from build123d import *

# Parameters (mm, degrees)
SALIENTE_EXTRUIR1_DEPTH = 2
SALIENTE_EXTRUIR2_DEPTH = 100
CROQUIS3_W              = 58.7
CROQUIS3_H              = 38.2
CROQUIS3_R              = 1.5
CROQUIS3_W_2            = 38.8
CROQUIS3_H_2            = 35.8
CORTAR_EXTRUIR1_DEPTH   = 1
CROQUIS4_W              = 38.8
CROQUIS4_H              = 35.8
CORTAR_EXTRUIR2_DEPTH   = 12
CROQUIS5_W              = 58.7
CROQUIS5_H              = 38.2
CROQUIS5_R              = 1.5
CORTAR_EXTRUIR3_DEPTH   = 3
CROQUIS6_R              = 1
SALIENTE_EXTRUIR3_DEPTH = 3.4
CROQUIS8_R              = 1
CORTAR_EXTRUIR5_DEPTH   = 4
CORTAR_EXTRUIR6_DEPTH   = 0.6


with BuildPart() as part:
    # Croquis1 → Saliente-Extruir1 (new body)
    with BuildSketch(Plane(origin=(0, 0, 0), x_dir=(1, 0, 0), z_dir=(0, 1, 0))):
        with BuildLine():
            Line((-121.24355653, -10), (-69.282032303, -100))
            ThreePointArc((-69.282032303, -100), (-61.961524227, -107.320508076), (-51.961524227, -110))
            Line((-51.961524227, -110), (51.961524227, -110))
            ThreePointArc((51.961524227, -110), (61.961524227, -107.320508076), (69.282032303, -100))
            Line((69.282032303, -100), (121.24355653, -10))
            ThreePointArc((121.24355653, -10), (123.923048454, 0), (121.24355653, 10))
            Line((121.24355653, 10), (69.282032303, 100))
            ThreePointArc((69.282032303, 100), (61.961524227, 107.320508076), (51.961524227, 110))
            Line((51.961524227, 110), (-51.961524227, 110))
            ThreePointArc((-51.961524227, 110), (-61.961524227, 107.320508076), (-69.282032303, 100))
            Line((-69.282032303, 100), (-121.24355653, 10))
            ThreePointArc((-121.24355653, 10), (-123.923048454, 0), (-121.24355653, -10))
        make_face()
    extrude(amount=SALIENTE_EXTRUIR1_DEPTH)

    # Croquis2 → Saliente-Extruir2 (add)
    with BuildSketch(Plane(origin=(0, 2, 0), x_dir=(1, 0, 0), z_dir=(0, 1, 0))):
        with BuildLine():
            Line((-69.282032303, 100), (-121.24355653, 10))
            ThreePointArc((-121.24355653, 10), (-123.923048454, 0), (-121.24355653, -10))
            Line((-121.24355653, -10), (-69.282032303, -100))
            ThreePointArc((-69.282032303, -100), (-61.961524227, -107.320508076), (-51.961524227, -110))
            Line((-51.961524227, -110), (51.961524227, -110))
            ThreePointArc((51.961524227, -110), (61.961524227, -107.320508076), (69.282032303, -100))
            Line((69.282032303, -100), (121.24355653, -10))
            ThreePointArc((121.24355653, -10), (123.923048454, 0), (121.24355653, 10))
            Line((121.24355653, 10), (69.282032303, 100))
            ThreePointArc((69.282032303, 100), (61.961524227, 107.320508076), (51.961524227, 110))
            Line((51.961524227, 110), (-51.961524227, 110))
            ThreePointArc((-51.961524227, 110), (-61.961524227, 107.320508076), (-69.282032303, 100))
        make_face()
        with BuildLine():
            Line((-64.951905284, 97.5), (-116.913429511, 7.5))
            ThreePointArc((-116.913429511, 7.5), (-118.923048454, 0), (-116.913429511, -7.5))
            Line((-116.913429511, -7.5), (-64.951905284, -97.5))
            ThreePointArc((-64.951905284, -97.5), (-59.461524227, -102.990381057), (-51.961524227, -105))
            Line((-51.961524227, -105), (51.961524227, -105))
            ThreePointArc((51.961524227, -105), (59.461524227, -102.990381057), (64.951905284, -97.5))
            Line((64.951905284, -97.5), (116.913429511, -7.5))
            ThreePointArc((116.913429511, -7.5), (118.923048454, 0), (116.913429511, 7.5))
            Line((116.913429511, 7.5), (64.951905284, 97.5))
            ThreePointArc((64.951905284, 97.5), (59.461524227, 102.990381057), (51.961524227, 105))
            Line((51.961524227, 105), (-51.961524227, 105))
            ThreePointArc((-51.961524227, 105), (-59.461524227, 102.990381057), (-64.951905284, 97.5))
        make_face(mode=Mode.SUBTRACT)
    extrude(amount=SALIENTE_EXTRUIR2_DEPTH)

    # Croquis3 → Cortar-Extruir1 (cut)
    with BuildSketch(Plane(origin=(90.932667397, 0, 52.5), x_dir=(-0.49999999999999983, 0, 0.8660254037844387), z_dir=(-0.8660254037844387, 0, -0.49999999999999983))):
        with Locations((-1.426190801, 41.535179267)):
            Rectangle(CROQUIS3_W, CROQUIS3_H)
        with Locations((24.923809199, 57.635179267)):
            Circle(CROQUIS3_R, mode=Mode.SUBTRACT)
        with Locations((24.923809199, 25.435179267)):
            Circle(CROQUIS3_R, mode=Mode.SUBTRACT)
        with Locations((-27.776190801, 25.435179267)):
            Circle(CROQUIS3_R, mode=Mode.SUBTRACT)
        with Locations((-27.776190801, 57.635179267)):
            Circle(CROQUIS3_R, mode=Mode.SUBTRACT)
        with Locations((-4.376190801, 41.535179267)):
            Rectangle(CROQUIS3_W_2, CROQUIS3_H_2, mode=Mode.SUBTRACT)
    extrude(amount=-CORTAR_EXTRUIR1_DEPTH, mode=Mode.SUBTRACT)

    # Croquis4 → Cortar-Extruir2 (cut)
    with BuildSketch(Plane(origin=(90.932667397, 0, 52.5), x_dir=(-0.49999999999999983, 0, 0.8660254037844387), z_dir=(-0.8660254037844387, 0, -0.49999999999999983))):
        with Locations((-4.376190801, 41.535179267)):
            Rectangle(CROQUIS4_W, CROQUIS4_H)
    extrude(amount=-CORTAR_EXTRUIR2_DEPTH, mode=Mode.SUBTRACT)

    # Croquis5 → Cortar-Extruir3 (cut)
    with BuildSketch(Plane(origin=(91.798692801, 0, 53), x_dir=(-0.5, 0, 0.8660254037844386), z_dir=(-0.8660254037844387, 0, -0.5000000000000001))):
        with Locations((-1.426190801, 41.535179267)):
            Rectangle(CROQUIS5_W, CROQUIS5_H)
        with Locations((24.923809199, 25.435179267)):
            Circle(CROQUIS5_R, mode=Mode.SUBTRACT)
        with Locations((24.923809199, 57.635179267)):
            Circle(CROQUIS5_R, mode=Mode.SUBTRACT)
        with Locations((-27.776190801, 57.635179267)):
            Circle(CROQUIS5_R, mode=Mode.SUBTRACT)
        with Locations((-27.776190801, 25.435179267)):
            Circle(CROQUIS5_R, mode=Mode.SUBTRACT)
    extrude(amount=-CORTAR_EXTRUIR3_DEPTH, mode=Mode.SUBTRACT)

    # Croquis6 → Saliente-Extruir3 (add)
    # profile 1 of 4: a face of its own
    with BuildSketch(Plane(origin=(94.396769013, 0, 54.5), x_dir=(-0.5000000000000001, 0, 0.8660254037844386), z_dir=(-0.8660254037844386, 0, -0.5000000000000001))):
        with BuildLine():
            Line((-30.776190801, 60.635179267), (-25.776190801, 60.635179267))
            Line((-25.776190801, 60.635179267), (-25.776190801, 56.635179267))
            ThreePointArc((-25.776190801, 56.635179267), (-26.06908402, 55.928072486), (-26.776190801, 55.635179267))
            Line((-26.776190801, 55.635179267), (-30.776190801, 55.635179267))
            Line((-30.776190801, 55.635179267), (-30.776190801, 60.635179267))
        make_face()
        with Locations((-27.776190801, 57.635179267)):
            Circle(CROQUIS6_R, mode=Mode.SUBTRACT)
    # profile 2 of 4: a face of its own
    with BuildSketch(Plane(origin=(94.396769013, 0, 54.5), x_dir=(-0.5000000000000001, 0, 0.8660254037844386), z_dir=(-0.8660254037844386, 0, -0.5000000000000001))):
        with BuildLine():
            Line((-30.776190801, 22.435179267), (-25.776190801, 22.435179267))
            Line((-25.776190801, 22.435179267), (-25.776190801, 26.435179267))
            ThreePointArc((-25.776190801, 26.435179267), (-26.06908402, 27.142286049), (-26.776190801, 27.435179267))
            Line((-26.776190801, 27.435179267), (-30.776190801, 27.435179267))
            Line((-30.776190801, 27.435179267), (-30.776190801, 22.435179267))
        make_face()
        with Locations((-27.776190801, 25.435179267)):
            Circle(CROQUIS6_R, mode=Mode.SUBTRACT)
    # profile 3 of 4: a face of its own
    with BuildSketch(Plane(origin=(94.396769013, 0, 54.5), x_dir=(-0.5000000000000001, 0, 0.8660254037844386), z_dir=(-0.8660254037844386, 0, -0.5000000000000001))):
        with BuildLine():
            Line((27.923809199, 22.435179267), (22.923809199, 22.435179267))
            Line((22.923809199, 22.435179267), (22.923809199, 26.435179267))
            ThreePointArc((22.923809199, 26.435179267), (23.216702418, 27.142286049), (23.923809199, 27.435179267))
            Line((23.923809199, 27.435179267), (27.923809199, 27.435179267))
            Line((27.923809199, 27.435179267), (27.923809199, 22.435179267))
        make_face()
        with Locations((24.923809199, 25.435179267)):
            Circle(CROQUIS6_R, mode=Mode.SUBTRACT)
    # profile 4 of 4: a face of its own
    with BuildSketch(Plane(origin=(94.396769013, 0, 54.5), x_dir=(-0.5000000000000001, 0, 0.8660254037844386), z_dir=(-0.8660254037844386, 0, -0.5000000000000001))):
        with BuildLine():
            Line((27.923809199, 60.635179267), (22.923809199, 60.635179267))
            Line((22.923809199, 60.635179267), (22.923809199, 56.635179267))
            ThreePointArc((22.923809199, 56.635179267), (23.216702418, 55.928072486), (23.923809199, 55.635179267))
            Line((23.923809199, 55.635179267), (27.923809199, 55.635179267))
            Line((27.923809199, 55.635179267), (27.923809199, 60.635179267))
        make_face()
        with Locations((24.923809199, 57.635179267)):
            Circle(CROQUIS6_R, mode=Mode.SUBTRACT)
    extrude(amount=SALIENTE_EXTRUIR3_DEPTH)

    # Croquis8 → Cortar-Extruir5 (cut)
    with BuildSketch(Plane(origin=(90.932667397, 0, 52.5), x_dir=(-0.49999999999999983, 0, 0.8660254037844387), z_dir=(-0.8660254037844387, 0, -0.49999999999999983))):
        with Locations((-27.776190801, 57.635179267)):
            Circle(CROQUIS8_R)
        with Locations((-27.776190801, 25.435179267)):
            Circle(CROQUIS8_R)
        with Locations((24.923809199, 25.435179267)):
            Circle(CROQUIS8_R)
        with Locations((24.923809199, 57.635179267)):
            Circle(CROQUIS8_R)
    extrude(amount=-CORTAR_EXTRUIR5_DEPTH, mode=Mode.SUBTRACT)

    # Croquis10 → Cortar-Extruir6 (cut)
    with BuildSketch(Plane(origin=(90.932667397, 0, 52.5), x_dir=(-0.49999999999999983, 0, 0.8660254037844387), z_dir=(-0.8660254037844387, 0, -0.49999999999999983))):
        Polygon((27.923809199, 22.435179267), (27.923809199, 60.635179267), (-30.776190801, 60.635179267), (-30.776190801, 55.635179267), (-30.776190801, 27.435179267), (-30.776190801, 22.435179267), align=None)
    extrude(amount=-CORTAR_EXTRUIR6_DEPTH, mode=Mode.SUBTRACT)


solid = part.part
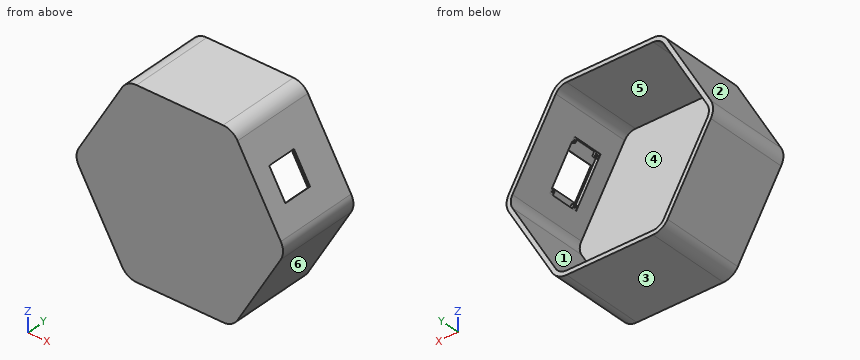
Model file for the job. Use its own axes, mm. Face numbers are marked on the shaded views. A direction names the side the tool comes from. Give positions to 0.01 mm unless a question says otherwise; leave off trailing zeros. Order: outer loops, then holes, each group sorted by start corner. A loop starts at its lowest first (then second) coordinate and runs counter-clockwise, first axis right, second up. Notation, with made-up numbers: M 44,41.5 L 92,41.5 A33 ccw 92,73.5 Z; hole C 75,48 d1. An arc over 180 degrees is marked long. Write item = value, one per line.
Q1. Flat gauge pins, fed straight in: pin 1 (9 mm diameter, centred on x = 87, z = 44, fed in from +Y); pin 2 (3 mm diameter, centred on x = 73.5, y = 11, fed in from -Z). Where does each tip first touch, or does it go through?
Derived:
pin_1 = 2
pin_2 = -95.29
Q2. Tool access for the marked faces 5 and 6: list every direction of +Z, -Z, +X, -X, +Y, -Y with a clear straight run to the whole face (end or side of a thin tool).
Derived:
face_5 = +Y
face_6 = -Z, +X, +Y, -Y
Q3. Drill centre lines: line 1 (Z direction, x = -48.5, y = 42); line 2 (X direction, y = 30.5, z = 77); line 3 (Y direction, x = 19.5, z = 13). Where is each one in solid material? Low to high. Write a range as [from, to].
Derived:
line_1 = [-110, -105], [105, 110]
line_2 = [-82.56, -76.79], [76.79, 77.52], [81.41, 82.56]
line_3 = [0, 2]
Q4. Cut at A-A, the plane y = 79. List the corners of the cut face in (x, z).
Derived:
outline = M -121.24,-10 L -69.28,-100 A20 ccw -51.96,-110 L 51.96,-110 A20 ccw 69.28,-100 L 121.24,-10 A20 ccw 121.24,10 L 69.28,100 A20 ccw 51.96,110 L -51.96,110 A20 ccw -69.28,100 L -121.24,10 A20 ccw Z; hole M -116.91,-7.5 L -64.95,-97.5 A15 ccw -51.96,-105 L 51.96,-105 A15 ccw 64.95,-97.5 L 116.91,-7.5 A15 ccw 116.91,7.5 L 64.95,97.5 A15 ccw 51.96,105 L -51.96,105 A15 ccw -64.95,97.5 L -116.91,7.5 A15 ccw Z
Q5. Cut at B-B, the plane x = -13.5. List the corners of the cut face in (y, z), then the cut area to 3 significant figures.
Derived:
outline = M 0,-110 L 102,-110 L 102,-105 L 2,-105 L 2,105 L 102,105 L 102,110 L 0,110 Z
area = 1,440 mm2
Q6. Cut at C-C, the plane z = 52. List the corners of the cut face in (x, y).
Derived:
outline = M -96.99,0 L 96.99,0 L 96.99,23.64 L 95.84,23.64 L 95.84,22.44 L 91.22,22.44 L 91.22,2 L -91.22,2 L -91.22,102 L -96.99,102 Z; M 91.22,60.64 L 95.84,60.64 L 95.84,59.44 L 96.99,59.44 L 96.99,102 L 91.22,102 Z
Q7. Two-plate mould, pull along Z, no slides. Class the marked faces 1, 2, 3 and 4: pulls with the +Z half, pulls with the -Z half, needs draft (parallel to the pull), parting line crosses it, or undercut.
Derived:
face_1 = undercut
face_2 = pulls with the +Z half
face_3 = pulls with the -Z half
face_4 = undercut
